from build123d import *

# Parameters (mm, degrees)
F1_DEPTH  = 19.05
F0_R      = 63.5
F2_DEPTH  = 76.2
F0_R_2    = 31.75
F3_DEPTH  = 19.05
F0_R_3    = 19.05
F0_R_4    = 6.35
F4_DEPTH  = 50.8
F5_R      = 19.05
F6_DEPTH  = 12.7
F7_DEPTH  = 76.201
F8_DEPTH  = 19.05
F9_R      = 19.04999
F10_R     = 9.525
F11_DEPTH = 19.05


# Not quite as in the source:
# - a fillet or chamfer is up to 0.001 mm smaller than in the source, because OpenCascade refuses the exact size


with BuildPart() as f1:
    # F0 (on Top) → F1 (new body)
    with BuildSketch(Plane.XY):
        with BuildLine():
            ThreePointArc((0, 76.2), (53.8815367264, 53.8815367264), (76.2, 0))
            ThreePointArc((76.2, 0), (53.8815367264, -53.8815367264), (0, -76.2))
            Line((0, -76.2), (127, -76.2))
            Line((127, -76.2), (127, -38.1))
            Line((127, -38.1), (88.9, -38.1))
            Line((88.9, -38.1), (88.9, 38.1))
            Line((88.9, 38.1), (127, 38.1))
            Line((127, 38.1), (127, 76.2))
            Line((127, 76.2), (0, 76.2))
        make_face()
    extrude(amount=F1_DEPTH)

    # F0 (on Top) → F2 (join)
    with BuildSketch(Plane.XY):
        with BuildLine():
            ThreePointArc((0, -76.2), (53.8815367264, -53.8815367264), (76.2, 0))
            ThreePointArc((76.2, 0), (53.8815367264, 53.8815367264), (0, 76.2))
            ThreePointArc((0, 76.2), (-76.2, 0), (0, -76.2))
        make_face()
        Circle(F0_R, mode=Mode.SUBTRACT)
    extrude(amount=F2_DEPTH)

    # F0 (on Top) → F3 (join)
    with BuildSketch(Plane.XY):
        Circle(F0_R)
        Circle(F0_R_2, mode=Mode.SUBTRACT)
    extrude(amount=F3_DEPTH)

    # F0 (on Top) → F4 (join)
    with BuildSketch(Plane.XY):
        Circle(F0_R_2)
        Circle(F0_R_3, mode=Mode.SUBTRACT)
        Circle(F0_R_3)
        Circle(F0_R_4, mode=Mode.SUBTRACT)
        Circle(F0_R_4)
    extrude(amount=F4_DEPTH)

    # F5 (on face) → F6 (cut)
    with BuildSketch(Plane.XY.offset(50.8)):
        Circle(F5_R)
    extrude(amount=-F6_DEPTH, mode=Mode.SUBTRACT)

    # F0 (on Top) → F7 (cut, through all)
    with BuildSketch(Plane.XY):
        Circle(F0_R_4)
    extrude(amount=F7_DEPTH, mode=Mode.SUBTRACT)

    # F0 (on Top) → F8 (join)
    with BuildSketch(Plane.XY):
        with BuildLine():
            ThreePointArc((0, -76.2), (-76.2, 0), (0, 76.2))
            Line((0, 76.2), (-127, 76.2))
            Line((-127, 76.2), (-127, 38.1))
            Line((-127, 38.1), (-88.9, 38.1))
            Line((-88.9, 38.1), (-88.9, -38.1))
            Line((-88.9, -38.1), (-127, -38.1))
            Line((-127, -38.1), (-127, -76.2))
            Line((-127, -76.2), (0, -76.2))
        make_face()
    extrude(amount=F8_DEPTH)

    # F9 (radius 19.05 in the source; OpenCascade refuses exactly that, so slightly less here)
    f9_edges = [f1.edges().sort_by_distance(p)[0] for p in [
        (-127, -76.2, 9.525),
        (-127, -38.1, 9.525),
        (-127, 38.1, 9.525),
        (-127, 76.2, 9.525),
        (127, 38.1, 9.525),
        (127, 76.2, 9.525),
        (127, -76.2, 9.525),
        (127, -38.1, 9.525),
    ]]
    fillet(f9_edges, radius=F9_R)

    # F10 (on face) → F11 (cut, through all)
    with BuildSketch(Plane.XY.offset(19.05)):
        with Locations((-107.95, -57.15)):
            Circle(F10_R)
        with Locations((-107.95, 57.15)):
            Circle(F10_R)
        with Locations((107.95, 57.15)):
            Circle(F10_R)
        with Locations((107.95, -57.15)):
            Circle(F10_R)
    extrude(amount=-F11_DEPTH, mode=Mode.SUBTRACT)


solid = f1.part
Geometry: final body of the model. Coordinates: model frame, mm. A direction names the side the tool comes from. Give positions to 0.01 mm unless a question says otherwise; leave off trailing zeros. Write each loop counter-clockwise with the first axis right and the second up, starting at its lowest first coordinate (ties: lowest second). Pieces come first, ordered by that corner, then holes. Notation, with made-up numbers: (52, 44.5) - (86, 44.5) arc R13 ccw to (86, 58.5) - close; hole circle Ø7 at (44.25, 41.25). An arc over 180 degrees is marked (long way). Return JSON: item names as keys, results as strings. Group by question number.
1) First-contact query: P1, Ø25, axis at x = -107.95, y = 57.15, coming from the +Z side; P2, Ø9.5, axis at y = -19, z = 14, coming from the +X side; P3, Ø5, axis at y = 54, z = 28.5, coming from the -X side; P4, Ø15, axis at x = 107.95, y = -57.15, coming from the +Z side. Flat tips, straight axial feed; report the tip coordinate or a pass-through.
2) Line query: line 1 (Y direction, x = -107, z = 11); line 2 (X direction, y = 57, z = 14); line 3 (X direction, y = 4, z = 50). Output: solid intervals per line, ascending.
3) Mould query, pull axis Y, two halves, no side actions, for faces 1 (the flat face through (82, 0, 19.05)), 2 (the cylindrical face through (-60.47, -46.367, 47.225)), 3 (the flat face through (14, -14, 50.8)), 4 (the cylindrical face through (-121.27, -70.77, 9.66)). Classes: released by +Y, released by -Y, zero draft, split by the parting line, or undercut.
4) Set-up query: faces 5 (the flat face through (-2, -16, 0)), 6 (the flat face through (-99, 38.1, 9)), 7 (the flat face through (88.9, -1, 9)), 8 (the cylindrical face through (-13.77, -61.99, 47.22)), 9 (the cylindrical face through (-115.509, 51.354, 9.658)). Return all of +Z, -Z, +X, -X, +Y, -Y with unobstructed straight access to the full face (end or side cutting, diameter ignored); none if empty.
5) Section B-B on y = 61. Return the cut outline in (x, z), plus the area to 3 significant figures.
6) Section C-C on z = 45.5. Return the cut outline in (x, y).
7) Section D-D on z = 6. State how many separate pieces and enclosed holes the cut face has, plus the area to 3 significant figures.
8) Section A-A on y = 0. Return the cut outline in (x, z), plus the area to 3 significant figures.
Filled in:
{
 "1": {"P1": "stops at z = 19.05", "P2": "stops at x = 88.9", "P3": "stops at x = -56.16", "P4": "passes through"},
 "2": {"line 1": "y = -76.2 to -66.63, -47.67 to -38.1, 38.1 to 47.67, 66.63 to 76.2", "line 2": "x = -127 to -117.47, -98.43 to 98.43, 117.47 to 127", "line 3": "x = -76.09 to -63.37, -31.5 to -18.63, 18.63 to 31.5, 63.37 to 76.09"},
 "3": {"face 1": "zero draft", "face 2": "split by the parting line", "face 3": "undercut", "face 4": "released by -Y"},
 "4": {"face 5": "-Z, +X, -X, +Y, -Y", "face 6": "+Z, -Z, -X", "face 7": "+Z, -Z, +X", "face 8": "+Z", "face 9": "+Z, -Z"},
 "5": {"outline": "(-126.61, 0) - (-116.66, 0) - (-116.66, 19.05) - (-126.61, 19.05) - close; (-99.24, 0) - (99.24, 0) - (99.24, 19.05) - (45.67, 19.05) - (45.67, 76.2) - (17.64, 76.2) - (17.64, 19.05) - (-17.64, 19.05) - (-17.64, 76.2) - (-45.67, 76.2) - (-45.67, 19.05) - (-99.24, 19.05) - close; (116.66, 0) - (126.61, 0) - (126.61, 19.05) - (116.66, 19.05) - close", "area": "7,360 mm^2"},
 "6": {"outline": "circle Ø152.4 at (0, 0); circle Ø63.5 at (0, 0); hole circle Ø127 at (0, 0); hole circle Ø38.1 at (0, 0)"},
 "7": {"separate pieces": "1", "enclosed holes": "5", "area": "31,000 mm^2"},
 "8": {"outline": "(-88.9, 0) - (-6.35, 0) - (-6.35, 38.1) - (-19.05, 38.1) - (-19.05, 50.8) - (-31.75, 50.8) - (-31.75, 19.05) - (-63.5, 19.05) - (-63.5, 76.2) - (-76.2, 76.2) - (-76.2, 19.05) - (-88.9, 19.05) - close; (6.35, 0) - (88.9, 0) - (88.9, 19.05) - (76.2, 19.05) - (76.2, 76.2) - (63.5, 76.2) - (63.5, 19.05) - (31.75, 19.05) - (31.75, 50.8) - (19.05, 50.8) - (19.05, 38.1) - (6.35, 38.1) - close", "area": "5,890 mm^2"}
}
